The listing builds one solid part. Answer for the finished solid, in the listing's coordinates (mm). A direction names the side the tool comes from. Give positions to 0.01 mm unless a question says otherwise; leave off trailing zeros. Write each loop counter-clockwise with the first axis right and the second up, starting at its lowest first coordinate (ties: lowest second). Pieces come first, ordered by that corner, then holes. Notation, with made-up numbers: (23, 11) - (62, 11) arc R21 ccw to (62, 42) - close; hole circle Ø10 at (70, 0.25). An arc over 180 degrees is marked (long way). Answer as CSV lines item,"result". Start each with the question number.
(1) Find section B-B (x = 7). Write down the section's boundary in (y, z), then the cut area to 3 significant figures.
(2) For faces 4 (the face through (8, 4, -11)), 5 (the face through (4, 0.5, -11)), 6 (the face through (4, 8, -11)), 7 (the face through (0.5, 4, -11)), determine the directions among +Z, -Z, +X, -X, +Y, -Y from which every point of the face is accessible in a straight line to the end or side of a thin tool.
(3) Find section C-C (z = -15.5). Write down the section's boundary in (x, y).
(4) Find section D-D (y = 1.25). Write down the section's boundary in (x, z).
(5) For a pull along Y with two mould halves and no side action, classify faces 1 (the face through (4, 0, 1)), 2 (the face through (4.3, 7.51, -22.13)), 3 (the face through (0, 4, 1)) as pulls with the +Y half, pulls with the -Y half, needs draft (parallel to the pull), parting line crosses it, or undercut.
(6) Find section A-A (y = 7.5). Write down the section's boundary in (x, z), then the cut area to 3 significant figures.
(7) Each of these flat-tipped pins is pushed along its axis until it touches: pin 1 Ø1 at (x, z) = (6, -1.5) entering from -Y; pin 2 Ø1.5 at (x, y) = (3.5, 2.5) entering from -Z; pin 3 Ø1.5 at (y, z) = (7, -12) entering from +X; pin 4 Ø4 at (x, y) = (1.5, 6) entering from -Z. Where does it stop, or does it pass through?
(8) Straight lines are drawn through the part: probe 1 along Y at (x, z) = (4.25, -11.75); probe 2 along Z at (x, y) = (2.5, 2). For each, find the intervals that lie inside material, in ascending order.
from build123d import *

# Parameters (mm, degrees)
BOSS_EXTRUDE1_START   = -0.5
BOSS_EXTRUDE1_DEPTH   = 8
BOSS_EXTRUDE1_2_DEPTH = 7.5
CUT_EXTRUDE1_DEPTH    = 0.5
SKETCH3_W             = 8
SKETCH3_H             = 24.267949192
BOSS_EXTRUDE2_DEPTH   = 0.5
CUT_EXTRUDE2_DEPTH    = 7.5
CUT_EXTRUDE3_DEPTH    = 0.433012702
CUT_EXTRUDE4_DEPTH    = 20.834936491
SKETCH7_W             = 3
SKETCH7_H             = 8.5
BOSS_EXTRUDE3_DEPTH   = 0.5


with BuildPart() as part:
    # Boss-Extrude1: read off the stored shape, not the designer's step
    # Boss-Extrude1 outline → Boss-Extrude1 (new body)
    with BuildSketch(Plane.ZY.offset(-8).offset(BOSS_EXTRUDE1_START)):
        with BuildLine():
            Line((-21.267949192, 8.5), (-21.267949192, 3.5))
            Line((-21.267949192, 3.5), (-22.133974596, 2))
            ThreePointArc((-22.133974596, 2), (-22.133974596, 1), (-21.267949192, 0.5))
            Line((-21.267949192, 0.5), (3, 0.5))
            Line((3, 0.5), (3, 8.5))
            Line((3, 8.5), (-21.267949192, 8.5))
        make_face()
    extrude(amount=BOSS_EXTRUDE1_DEPTH)

    # Boss-Extrude1 2 outline → Boss-Extrude1 2 (add)
    with BuildSketch(Plane.ZY.offset(-8)):
        with BuildLine():
            Line((-22.133974596, 6.5), (-21.267949192, 5))
            Line((-21.267949192, 5), (-21.267949192, 8))
            ThreePointArc((-21.267949192, 8), (-22.133974596, 7.5), (-22.133974596, 6.5))
        make_face()
    extrude(amount=BOSS_EXTRUDE1_2_DEPTH)

    # Sketch2 → Cut-Extrude1 (cut)
    with BuildSketch(Plane(origin=(8.5, 0, 0), x_dir=(0, 0, -1), z_dir=(1, 0, 0))):
        with BuildLine():
            Line((22.133974596, 2), (21.267949192, 3.5))
            Line((21.267949192, 3.5), (21.267949192, 0.5))
            ThreePointArc((21.267949192, 0.5), (22.133974596, 1), (22.133974596, 2))
        make_face()
    extrude(amount=-CUT_EXTRUDE1_DEPTH, mode=Mode.SUBTRACT)

    # Sketch3 → Boss-Extrude2 (add)
    with BuildSketch(Plane.XZ.offset(-0.5)):
        with Locations((4.5, -9.133974596)):
            Rectangle(SKETCH3_W, SKETCH3_H)
    extrude(amount=BOSS_EXTRUDE2_DEPTH)

    # Sketch4 → Cut-Extrude2 (cut)
    with BuildSketch(Plane.ZY.offset(-0.5)):
        Polygon((-21.267949192, 3.5), (-20.834936491, 4.25), (-21.267949192, 5), align=None)
    extrude(amount=-CUT_EXTRUDE2_DEPTH, mode=Mode.SUBTRACT)

    # Sketch5 → Cut-Extrude3 (cut)
    with BuildSketch(Plane(origin=(0, 0, -21.267949192), x_dir=(-1, 0, 0), z_dir=(0, 0, -1))):
        Polygon((-0.5, 8), (-0.5, 8.5), (-8.5, 8.5), (-8.5, 0), (-0.5, 0), (-0.5, 0.5), (-8, 0.5), (-8, 4.25), (-8, 8), align=None)
    extrude(amount=-CUT_EXTRUDE3_DEPTH, mode=Mode.SUBTRACT)

    # Sketch6 → Cut-Extrude4 (cut)
    with BuildSketch(Plane(origin=(0, 0, -20.834936491), x_dir=(-1, 0, 0), z_dir=(0, 0, -1))):
        Polygon((-0.5, 8), (-0.5, 8.5), (-8.5, 8.5), (-8.5, 0), (-0.5, 0), (-0.5, 0.5), (-8, 0.5), (-8, 8), align=None)
    extrude(amount=-CUT_EXTRUDE4_DEPTH, mode=Mode.SUBTRACT)

    # Sketch7 → Boss-Extrude3 (add)
    with BuildSketch(Plane.ZY.offset(-0.5)):
        with Locations((1.5, 4.25)):
            Rectangle(SKETCH7_W, SKETCH7_H)
    extrude(amount=BOSS_EXTRUDE3_DEPTH)


solid = part.part
Result set:
1,outline,"(0, 0) - (0.5, 0) - (0.5, -21.27) arc R1 ccw to (2, -22.13) - (4.25, -20.83) - (6.5, -22.13) arc R1 ccw to (8, -21.27) - (8, 0) - (8.5, 0) - (8.5, 3) - (0, 3) - close"
1,area,"189 mm^2"
2,face 4,"-Z, +X, +Y, -Y"
2,face 5,"-Z, +X, -X, -Y"
2,face 6,"-Z, +X, -X, +Y"
2,face 7,"-Z, -X, +Y, -Y"
3,outline,"(0.5, 0.5) - (8, 0.5) - (8, 8) - (0.5, 8) - close"
4,outline,"(0, 0) - (0.5, 0) - (0.5, -22.24) - (8, -22.24) - (8, 0) - (8.5, 0) - (8.5, 3) - (0, 3) - close"
5,face 1,"pulls with the -Y half"
5,face 2,"undercut"
5,face 3,"needs draft"
6,outline,"(0, 0) - (0.5, 0) - (0.5, -22.13) - (8, -22.13) - (8, 0) - (8.5, 0) - (8.5, 3) - (0, 3) - close"
6,area,"192 mm^2"
7,pin 1,"y = 0.5"
7,pin 2,"z = -22.24"
7,pin 3,"x = 8"
7,pin 4,"z = -22.27"
8,probe 1,"0.5 to 8"
8,probe 2,"-22.13 to 3"
